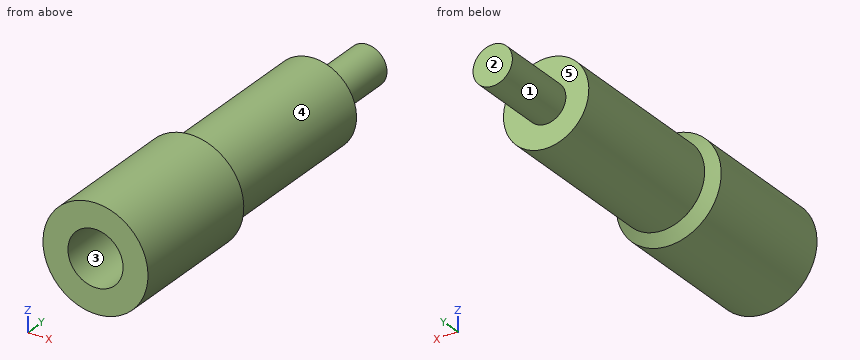
from build123d import *

# Parameters (mm, degrees)
SKETCH_1_R             = 4
EXTRUDE_1_DEPTH        = 24.5
SKETCH_2_R             = 1.5
EXTRUDE_2_DEPTH        = 6
HOLE_WIZARD_M5_1_D     = 4.2
HOLE_WIZARD_M5_1_DEPTH = 10
HOLE_WIZARD_M5_1_TIP   = 1.2618073
SKETCH_5_OUTSIDE_W     = 16.506
SKETCH_5_OUTSIDE_H     = 16.506
SKETCH_5_OUTSIDE_R     = 3.25
CUT_EXTRUDE_1_DEPTH    = 13
CHAMFER_1_SIZE         = 0.75


with BuildPart() as part:
    # 草图1 → 凸台-拉伸1 (new body)
    with BuildSketch(Plane(origin=(0, 0, 0), x_dir=(1, 0, 0), z_dir=(0, 1, 0))):
        with Locations(Location((0, 0, 0), (0, 0, 270))):
            Circle(SKETCH_1_R)
    extrude(amount=EXTRUDE_1_DEPTH)

    # 草图2 → 凸台-拉伸2 (add)
    with BuildSketch(Plane(origin=(0, 24.5, 0), x_dir=(1, 0, 0), z_dir=(0, 1, 0))):
        with Locations(Location((0, 0, 0), (0, 0, 270))):
            Circle(SKETCH_2_R)
    extrude(amount=EXTRUDE_2_DEPTH)

    # M5 螺纹孔1
    with Locations(Plane(origin=(0, 0, 0), x_dir=(-1, 0, 0), z_dir=(0, -1, 0))):
        with Locations((0, 0)):
            Hole(HOLE_WIZARD_M5_1_D / 2, depth=HOLE_WIZARD_M5_1_DEPTH)
            with Locations((0, 0, -(HOLE_WIZARD_M5_1_DEPTH + HOLE_WIZARD_M5_1_TIP / 2))):  # 118° drill point
                Cone(0, HOLE_WIZARD_M5_1_D / 2, HOLE_WIZARD_M5_1_TIP, mode=Mode.SUBTRACT)

    # 草图5 outside → 切除-拉伸1 (cut)
    with BuildSketch(Plane(origin=(0, 24.5, 0), x_dir=(1, 0, 0), z_dir=(0, 1, 0))):
        Rectangle(SKETCH_5_OUTSIDE_W, SKETCH_5_OUTSIDE_H)
        with Locations(Location((0, 0, 0), (0, 0, 270))):
            Circle(SKETCH_5_OUTSIDE_R, mode=Mode.SUBTRACT)
    extrude(amount=-CUT_EXTRUDE_1_DEPTH, mode=Mode.SUBTRACT)

    # 倒角1
    chamfer_1_edges = [part.edges().sort_by_distance(p)[0] for p in [
        (0, 11.5, -4),
    ]]
    chamfer(chamfer_1_edges, length=CHAMFER_1_SIZE - 0.0001)  # a hair under: the kernel refuses the full size


solid = part.part
Part model, mm, in its own coordinate system. Face numbers are marked on the shaded views. A direction names the side the tool comes from. Coordinates: 2 decimals unless noted, no trailing zeros. Order: outer loops, then holes, each group sorted by start corner. A loop starts at its lowest first (then second) coordinate and runs counter-clockwise, first axis right, second up. Notation, with made-up numbers: (3, 48.5) - (51, 48.5) arc R16 cw to (51, 71.5) - close; hole circle Ø5 at (-0.75, -38.5). An arc over 180 degrees is marked (long way). Use CSV: the item, a comma, the result in double quotes.
Item 1: Probe probe 1 along Z at (x, y) = (0, 3.75); probe 2 along Z at (x, y) = (0.75, 9); probe 3 along Y at (x, z) = (-2.5, -0.5). List the from-to ranges inside material, lowest first.
Solved:
probe 1,"z = -4 to -2.1, 2.1 to 4"
probe 2,"z = -3.93 to -1.96, 1.96 to 3.93"
probe 3,"y = 0 to 24.5"
Item 2: 3-axis set-ups, long thin cutter, end or side, ignore diameter. For the marked faces 1 and 2: which of +Z, -Z, +X, -X, +Y, -Y reach the whole face in a straight line?
Solved:
face 1,"+Y"
face 2,"+Z, -Z, +X, -X, +Y"
Item 3: Mould opens along X. For the marked faces 3, 4 and 5 say: +X half, -X half, draft (parallel to the pull), parting line (faces both ways), or undercut.
Solved:
face 3,"undercut"
face 4,"parting line"
face 5,"draft"
Item 4: Drop flat-ended pins along their axis: P1, Ø2, axis at x = -3, y = 5.5, coming from the +Z side; P2, Ø1.5, axis at x = -0.5, z = 1.5, coming from the +Y side. Give the stop position or say it passes through.
Solved:
P1,"stops at z = 3.46"
P2,"stops at y = 30.5"
Item 5: Saw through at A-A on y = 9. Give the cut face in (x, z), and give its area (3 significant figures).
Solved:
outline,"circle Ø8 at (0, 0); hole circle Ø4.2 at (0, 0)"
area,"36.4 mm²"
Item 6: Saw through at B-B on y = 29. Give the cut face in (x, z).
Solved:
outline,"circle Ø3 at (0, 0)"
Item 7: Saw through at C-C on y = 16.5. Give the cut face in (x, z), and give its area (3 significant figures).
Solved:
outline,"circle Ø6.5 at (0, 0)"
area,"33.2 mm²"
